Verification items for the finished model (mm, model axes). A direction names the side the tool comes from. Round coordinates to 2 decimals unless told otherwise and drop trailing zeros. Write each loop counter-clockwise with the first axis right and the second up, starting at its lowest first coordinate (ties: lowest second). Pieces come first, ordered by that corner, then holes. Notation, with made-up numbers: (7.5, 30) - (53.5, 30) arc R16 ccw to (53.5, 38) - close; hole circle Ø6 at (71, -24). An arc over 180 degrees is marked (long way). Write each question's results on one line, items separated by ' | '.
```python
from build123d import *

# Parameters (mm, degrees)
F0_W     = 31.4
F0_H     = 7.4
F0_R     = 3
F1_DEPTH = 3.95
F0_R_2   = 2.499
F2_DEPTH = 2.95
F3_R     = 3.69999


# Not quite as in the source:
# - a fillet or chamfer is up to 0.001 mm smaller than in the source, because OpenCascade refuses the exact size


with BuildPart() as f1:
    # F0 (on Front) → F1 (new body, symmetric)
    with BuildSketch(Plane.XZ):
        Rectangle(F0_W, F0_H)
        with BuildLine():
            ThreePointArc((-12.9, 2.8618176043), (-12, 3), (-11.1, 2.8618176043))
            Line((-11.1, 2.8618176043), (-11.1, 0.9))
            Line((-11.1, 0.9), (-9.1381823957, 0.9))
            ThreePointArc((-9.1381823957, 0.9), (-9, 0), (-9.1381823957, -0.9))
            Line((-9.1381823957, -0.9), (-11.1, -0.9))
            Line((-11.1, -0.9), (-11.1, -2.8618176043))
            ThreePointArc((-11.1, -2.8618176043), (-12, -3), (-12.9, -2.8618176043))
            Line((-12.9, -2.8618176043), (-12.9, -0.9))
            Line((-12.9, -0.9), (-14.8618176043, -0.9))
            ThreePointArc((-14.8618176043, -0.9), (-15, 0), (-14.8618176043, 0.9))
            Line((-14.8618176043, 0.9), (-12.9, 0.9))
            Line((-12.9, 0.9), (-12.9, 2.8618176043))
        make_face(mode=Mode.SUBTRACT)
        with Locations((-4, 0)):
            Circle(F0_R, mode=Mode.SUBTRACT)
        with Locations((4, 0)):
            Circle(F0_R, mode=Mode.SUBTRACT)
        with Locations((12, 0)):
            Circle(F0_R, mode=Mode.SUBTRACT)
    extrude(amount=F1_DEPTH, both=True)

    # F0 (on Front) → F2 (join, symmetric)
    with BuildSketch(Plane.XZ):
        with Locations((-4, 0)):
            Circle(F0_R)
        with Locations((-4, 0)):
            Circle(F0_R_2, mode=Mode.SUBTRACT)
        with Locations((4, 0)):
            Circle(F0_R)
        with Locations((4, 0)):
            Circle(F0_R_2, mode=Mode.SUBTRACT)
        with Locations((12, 0)):
            Circle(F0_R)
        with Locations((12, 0)):
            Circle(F0_R_2, mode=Mode.SUBTRACT)
    extrude(amount=F2_DEPTH, both=True)

    # F3 (radius 3.7 in the source; OpenCascade refuses exactly that, so slightly less here)
    f3_edges = [f1.edges().sort_by_distance(p)[0] for p in [
        (-15.7, 0, 3.7),
        (-15.7, 0, -3.7),
        (15.7, 0, 3.7),
        (15.7, 0, -3.7),
    ]]
    fillet(f3_edges, radius=F3_R)


solid = f1.part
```
(1) Section check C-C (x = -12.5). Record the cut outline in (y, z).
Answer:
outline: (-3.95, -3.67) - (3.95, -3.67) - (3.95, -2.96) - (-3.95, -2.96) - close; (-3.95, 2.96) - (3.95, 2.96) - (3.95, 3.67) - (-3.95, 3.67) - close
(2) Go/stop test with flat-tipped pins: pin 1 Ø0.6 at (y, z) = (-1, -2.5) entering from -X; pin 2 Ø0.6 at (y, z) = (-0.5, 2.5) entering from +X; pin 3 Ø1.6 at (y, z) = (-0.5, -2) entering from +X. Record where each tip stops, or that it passes through.
Answer:
pin 1: x = -14.97 | pin 2: x = 14.97 | pin 3: x = 15.5
(3) Thickness scan on L1, parallel to Z at x = -4, y = 2.35; L2, parallel to Z at x = -11, y = 1; L3, parallel to X at y = 1.5, z = -0.5. Record the ranges inside material, lowest first.
Answer:
L1: -3.7 to -2.5, 2.5 to 3.7 | L2: -3.7 to -0.9, 0.9 to 3.7 | L3: -15.67 to -14.96, -9.04 to -6.45, -1.55 to 1.55, 6.45 to 9.55, 14.45 to 15.67
(4) Section check A-A (x = -4). Record the cut outline in (y, z), plus the area to 3 significant figures.
Answer:
outline: (-3.95, -3.7) - (3.95, -3.7) - (3.95, -3) - (2.95, -3) - (2.95, -2.5) - (-2.95, -2.5) - (-2.95, -3) - (-3.95, -3) - close; (-3.95, 3) - (-2.95, 3) - (-2.95, 2.5) - (2.95, 2.5) - (2.95, 3) - (3.95, 3) - (3.95, 3.7) - (-3.95, 3.7) - close | area: 17.0 mm2
(5) Mould release check, pull along X, two halves, no side actions. Record for faces 4 (the cylindrical face through (-15, 0, 0)), 5 (the flat face through (0, 0, 3.7)), 6 (the cylindrical face through (-14.64, -0.06, -2.59)): released by +X, released by -X, zero draft, split by the parting line, or undercut.
Answer:
face 4: undercut | face 5: zero draft | face 6: released by -X
(6) Section check B-B (y = -1.5). State how many separate pieces and enclosed holes the cut face has, plus the area to 3 significant figures.
Answer:
separate pieces: 1 | enclosed holes: 4 | area: 144 mm2
(7) Set-up check for faces 1 (the cylindrical face through (-1.14, 3.46, 0.9)), 2 (the cylindrical face through (-12, 0, -3)), 3 (the cylindrical face through (1, -3.4, 0.1)): record each of +Z, -Z, +X, -X, +Y, -Y from which the full face is reachable in a straight line by a thin tool's end or side.
Answer:
face 1: +Y | face 2: +Y, -Y | face 3: -Y
